```python
from build123d import *

# Parameters (mm, degrees)
F0_R     = 14.2875
F1_DEPTH = 41.148
F0_R_2   = 6.35
F2_DEPTH = 11.176
F4_DEPTH = 3.175


# Not quite as in the source:
# - a feature of the source that left no trace in its solid (it failed there, or was rolled back) is left out


with BuildPart() as f1:
    # F0 (on Top) → F1 (new body)
    with BuildSketch(Plane.XY):
        with BuildLine():
            ThreePointArc((23.3629201096, -9.9666425617), (24.8855195926, -5.0863458994), (25.4, 0))
            ThreePointArc((25.4, 0), (-5.0863458994, 24.8855195926), (-23.3629201096, -9.9666425617))
            ThreePointArc((-23.3629201096, -9.9666425617), (0, -25.4), (23.3629201096, -9.9666425617))
        make_face()
        Circle(F0_R, mode=Mode.SUBTRACT)
    extrude(amount=F1_DEPTH)

    # F0 (on Top) → F2 (join)
    with BuildSketch(Plane.XY):
        with BuildLine():
            ThreePointArc((-23.3629201096, -9.9666425617), (-5.0863458994, 24.8855195926), (25.4, 0))
            ThreePointArc((25.4, 0), (24.8855195926, -5.0863458994), (23.3629201096, -9.9666425617))
            Line((23.3629201096, -9.9666425617), (46.0971900822, 43.3250180788))
            ThreePointArc((46.0971900822, 43.3250180788), (44.4699820006, 61.3000974853), (28.575, 69.85))
            Line((28.575, 69.85), (-28.575, 69.85))
            ThreePointArc((-28.575, 69.85), (-44.4699820006, 61.3000974853), (-46.0971900822, 43.3250180788))
            Line((-46.0971900822, 43.3250180788), (-23.3629201096, -9.9666425617))
        make_face()
        with Locations((-28.575, 50.8)):
            Circle(F0_R_2, mode=Mode.SUBTRACT)
        with Locations((28.575, 50.8)):
            Circle(F0_R_2, mode=Mode.SUBTRACT)
    extrude(amount=F2_DEPTH)

    # F3 (on Right) → F4 (join, symmetric)
    with BuildSketch(Plane.YZ):
        Polygon((66.675, 11.176), (25.4, 35.0061323608), (25.4, 11.176), align=None)
        Polygon((25.4, 11.176), (25.4, 35.0061323608), (22.225, 36.8392194655), (22.225, 11.176), align=None)
    extrude(amount=F4_DEPTH, both=True)


solid = f1.part
```
Input: part model. Units: mm. Frame: model coordinates. A direction names the side the tool comes from. Coordinates: 2 decimals unless noted, no trailing zeros. Write each loop counter-clockwise with the first axis right and the second up, starting at its lowest first coordinate (ties: lowest second). Pieces come first, ordered by that corner, then holes. Notation, with made-up numbers: (15, -1.75) - (55, -1.75) arc R24 ccw to (55, 17.25) - close; hole circle Ø11 at (22, 39). An arc over 180 degrees is marked (long way). Put each result on its own line as item: value. Start each with the question number.
1) Cut plane D-D (y = 3). Return the cut outline in (x, z), plus the area to 3 significant figures.
2) Cut plane C-C (y = 50.8). Return the cut outline in (x, z) (3 decimals), plus the area to 3 significant figures.
3) Ray query, L1, parallel to Y at x = 0, z = 11; L2, parallel to X at y = 50, z = 8; L3, parallel to Z at x = -35, y = 34. Return the intervals inside material, ascending.
4) Cut plane A-A (z = 7). State how many separate pieces and enclosed holes the cut face has, plus the area to 3 significant figures.
5) Cut plane B-B (x = 27). Return the cut outline in (y, z).
6) Mould query, pull axis Y, two halves, no side actions, for faces 3 (the face through (-34.89, 17.05, 5.51)), 4 (the face through (-3.175, 36, 18)), 5 (the face through (-22.52, 52.71, 5.51)). Classes: pulls with the +Y half, pulls with the -Y half, needs draft (parallel to the pull), parting line crosses it, or undercut.
7) Reachability of faces 1 (the face through (3.175, 36, 18)), 2 (the face through (11, -11, 41.148)) from +Z, -Z, +X, -X, +Y, -Y: full face, straight path, thin tool, end or side. Return the list, or none.
8) Contact query for flat-ended pins moving along their axis: pin 1 (7 mm diameter, centred on y = 48, z = 26.5, fed in from -X); pin 2 (3 mm diameter, centred on x = -20.5, z = 14, fed in from -Y); pin 3 (24 mm diameter, centred on x = -17, y = 45, fed in from +Z); pin 4 (5 mm diameter, centred on y = 42.5, z = 23.5, fed in from -X) (3 decimals). Output: stop coordinate, or through.
Resolved:
1. outline: (-28.89, 0) - (-13.97, 0) - (-13.97, 41.15) - (-25.22, 41.15) - (-25.22, 11.18) - (-28.89, 11.18) - close; (13.97, 0) - (28.89, 0) - (28.89, 11.18) - (25.22, 11.18) - (25.22, 41.15) - (13.97, 41.15) - close
1. area: 1,010 mm2
2. outline: (-47.625, 0) - (-34.925, 0) - (-34.925, 11.176) - (-47.625, 11.176) - close; (-22.225, 0) - (22.225, 0) - (22.225, 11.176) - (3.175, 11.176) - (3.175, 20.341) - (-3.175, 20.341) - (-3.175, 11.176) - (-22.225, 11.176) - close; (34.925, 0) - (47.625, 0) - (47.625, 11.176) - (34.925, 11.176) - close
2. area: 839 mm2
3. L1: y = -25.4 to -14.29, 14.29 to 69.85
3. L2: x = -47.61 to -34.87, -22.28 to 22.28, 34.87 to 47.61
3. L3: z = 0 to 11.18
4. separate pieces: 1
4. enclosed holes: 3
4. area: 5,690 mm2
5. outline: (-1.44, 0) - (44.65, 0) - (44.65, 11.18) - (-1.44, 11.18) - close; (56.95, 0) - (69.85, 0) - (69.85, 11.18) - (56.95, 11.18) - close
6. face 3: pulls with the -Y half
6. face 4: needs draft
6. face 5: undercut
7. face 1: +Z, +X, +Y
7. face 2: +Z, +X, -X, +Y, -Y
8. pin 1: passes through
8. pin 2: stops at y = -16.86
8. pin 3: stops at z = 11.18
8. pin 4: stops at x = -3.175
